```python
from build123d import *

# Parameters (mm, degrees)
SKETCH_1_W           = 46
SKETCH_1_H           = 30
EXTRUDE_1_DEPTH      = 3.5
SKETCH_2_W           = 46
SKETCH_2_H           = 5
EXTRUDE_2_DEPTH      = 33.5
SKETCH_4_R           = 1.3
CUT_EXTRUDE_2_DEPTH  = 15
SKETCH_5_R           = 1.3
CUT_EXTRUDE_3_DEPTH  = 15
CUT_EXTRUDE_4_REACH  = 49.71
SKETCH_6_W           = 5
SKETCH_6_H           = 3.7
SKETCH_7_W           = 46
SKETCH_7_H           = 25
EXTRUDE_3_DEPTH      = 15
SKETCH_8_W           = 46
SKETCH_8_H           = 2
CUT_EXTRUDE_5_DEPTH  = 14
SKETCH_10_W          = 5
SKETCH_10_H          = 3.7
CUT_EXTRUDE_7_DEPTH  = 5
FILLET_1_R           = 6
FILLET_2_R           = 4
SKETCH_11_W          = 5
SKETCH_11_H          = 23.135705429
CUT_EXTRUDE_8_DEPTH  = 14
FILLET_3_R           = 4
FILLET_4_R           = 1
SKETCH_12_W          = 1.2
SKETCH_12_H          = 0.5
EXTRUDE_4_DEPTH      = 10
SKETCH_13_W          = 1.2
SKETCH_13_H          = 0.5
EXTRUDE_5_DEPTH      = 10
SKETCH_14_W          = 57.080352076
SKETCH_14_H          = 14
CUT_EXTRUDE_9_DEPTH  = 2.5
FILLET_5_R           = 4
SKETCH_15_R          = 1.3
CUT_EXTRUDE_10_DEPTH = 8
SKETCH_16_W          = 5
SKETCH_16_H          = 1.8
CUT_EXTRUDE_11_DEPTH = 7
SKETCH_17_W          = 5
SKETCH_17_H          = 1.8
CUT_EXTRUDE_12_DEPTH = 7
SKETCH_18_R          = 3
CUT_EXTRUDE_13_DEPTH = 4


with BuildPart() as part:
    # Эскиз1 → Бобышка-Вытянуть1 (new body)
    with BuildSketch(Plane.XY):
        Rectangle(SKETCH_1_W, SKETCH_1_H)
    extrude(amount=EXTRUDE_1_DEPTH)

    # Эскиз2 → Бобышка-Вытянуть2 (add)
    with BuildSketch(Plane(origin=(0, 0, 0), x_dir=(-1, 0, 0), z_dir=(0, 0, -1))):
        with Locations((0, -12.5)):
            Rectangle(SKETCH_2_W, SKETCH_2_H)
    extrude(amount=EXTRUDE_2_DEPTH)

    # Эскиз4 → Вырез-Вытянуть2 (cut)
    with BuildSketch(Plane(origin=(0, 15, 0), x_dir=(1, 0, 0), z_dir=(0, 1, 0))):
        with Locations(Location((15, -1.5, 0), (0, 0, 270))):
            Circle(SKETCH_4_R)
        with Locations(Location((-15, -1.5, 0), (0, 0, 270))):
            Circle(SKETCH_4_R)
    extrude(amount=-CUT_EXTRUDE_2_DEPTH, mode=Mode.SUBTRACT)

    # Эскиз5 → Вырез-Вытянуть3 (cut)
    with BuildSketch(Plane(origin=(0, 0, -33.5), x_dir=(-1, 0, 0), z_dir=(0, 0, -1))):
        with Locations((-20, -12.5)):
            Circle(SKETCH_5_R)
        with Locations((20, -12.5)):
            Circle(SKETCH_5_R)
    extrude(amount=-CUT_EXTRUDE_3_DEPTH, mode=Mode.SUBTRACT)

    # Эскиз6 → Вырез-Вытянуть4 (cut, up to next)
    with BuildSketch(Plane(origin=(0, -10, 0), x_dir=(1, 0, 0), z_dir=(0, 1, 0)), mode=Mode.PRIVATE) as cut_extrude_4_sk1:
        with Locations((-15, 25.35)):
            Rectangle(SKETCH_6_W, SKETCH_6_H)
    cut_extrude_4_tool1 = extrude(cut_extrude_4_sk1.sketch, amount=-CUT_EXTRUDE_4_REACH, mode=Mode.PRIVATE) & part.part
    # Эскиз6 → Вырез-Вытянуть4 (cut, up to next)
    with BuildSketch(Plane(origin=(0, -10, 0), x_dir=(1, 0, 0), z_dir=(0, 1, 0)), mode=Mode.PRIVATE) as cut_extrude_4_sk2:
        with Locations((15, 25.35)):
            Rectangle(SKETCH_6_W, SKETCH_6_H)
    cut_extrude_4_tool2 = extrude(cut_extrude_4_sk2.sketch, amount=-CUT_EXTRUDE_4_REACH, mode=Mode.PRIVATE) & part.part
    add(cut_extrude_4_tool1.solids().sort_by_distance((-15, -10, -25.35))[0], mode=Mode.SUBTRACT)
    add(cut_extrude_4_tool2.solids().sort_by_distance((15, -10, -25.35))[0], mode=Mode.SUBTRACT)

    # Эскиз7 → Бобышка-Вытянуть3 (add)
    with BuildSketch(Plane(origin=(0, 0, 0), x_dir=(-1, 0, 0), z_dir=(0, 0, -1))):
        with Locations((0, 2.5)):
            Rectangle(SKETCH_7_W, SKETCH_7_H)
    extrude(amount=EXTRUDE_3_DEPTH)

    # Эскиз8 → Вырез-Вытянуть5 (cut)
    with BuildSketch(Plane(origin=(0, 0, -15), x_dir=(-1, 0, 0), z_dir=(0, 0, -1))):
        with Locations((0, 6.62)):
            Rectangle(SKETCH_8_W, SKETCH_8_H)
        with Locations((0, -1.38)):
            Rectangle(SKETCH_8_W, SKETCH_8_H)
    extrude(amount=-CUT_EXTRUDE_5_DEPTH, mode=Mode.SUBTRACT)

    # Эскиз10 → Вырез-Вытянуть7 (cut)
    with BuildSketch(Plane.XY.offset(3.5)):
        with Locations((15, 6)):
            Rectangle(SKETCH_10_W, SKETCH_10_H)
        with Locations((-15, 6)):
            Rectangle(SKETCH_10_W, SKETCH_10_H)
    extrude(amount=-CUT_EXTRUDE_7_DEPTH, mode=Mode.SUBTRACT)

    # Скругление1
    fillet_1_edges = [part.edges().sort_by_distance(p)[0] for p in [
        (0, -15, 3.5),
    ]]
    fillet(fillet_1_edges, radius=FILLET_1_R)

    # Скругление2
    fillet_2_edges = [part.edges().sort_by_distance(p)[0] for p in [
        (0, -10, -15),
    ]]
    fillet(fillet_2_edges, radius=FILLET_2_R)

    # Эскиз11 → Вырез-Вытянуть8 (cut)
    with BuildSketch(Plane(origin=(0, 0, -15), x_dir=(-1, 0, 0), z_dir=(0, 0, -1))):
        with Locations((0, -5.947852714)):
            Rectangle(SKETCH_11_W, SKETCH_11_H)
    extrude(amount=-CUT_EXTRUDE_8_DEPTH, mode=Mode.SUBTRACT)

    # Скругление3
    # the kernel refuses this fillet: 4 mm, written as the material it takes off along each edge
    with BuildSketch(Plane(origin=(-2.5, 5.62, -25), x_dir=(-1, 0, 0), z_dir=(0, 0, 1))) as fillet_3_piece_1:
        with BuildLine():
            CenterArc((FILLET_3_R, FILLET_3_R), FILLET_3_R, 180, 90)
            Line((0, FILLET_3_R), (0, 0))
            Line((0, 0), (FILLET_3_R, 0))
        make_face()
    extrude(amount=24, mode=Mode.SUBTRACT)
    with BuildSketch(Plane(origin=(-2.5, -2.38, -1), x_dir=(-1, 0, 0), z_dir=(0, 0, -1))) as fillet_3_piece_2:
        with BuildLine():
            CenterArc((FILLET_3_R, -FILLET_3_R), FILLET_3_R, 90, 90)
            Line((0, -FILLET_3_R), (0, 0))
            Line((0, 0), (FILLET_3_R, 0))
        make_face()
    extrude(amount=14, mode=Mode.SUBTRACT)
    with BuildSketch(Plane(origin=(2.5, -2.38, -15), x_dir=(0, -1, 0), z_dir=(0, 0, 1))) as fillet_3_piece_3:
        with BuildLine():
            CenterArc((FILLET_3_R, FILLET_3_R), FILLET_3_R, 180, 90)
            Line((0, FILLET_3_R), (0, 0))
            Line((0, 0), (FILLET_3_R, 0))
        make_face()
    extrude(amount=14, mode=Mode.SUBTRACT)
    with BuildSketch(Plane(origin=(2.5, 5.62, -25), x_dir=(1, 0, 0), z_dir=(0, 0, 1))) as fillet_3_piece_4:
        with BuildLine():
            CenterArc((FILLET_3_R, -FILLET_3_R), FILLET_3_R, 90, 90)
            Line((0, -FILLET_3_R), (0, 0))
            Line((0, 0), (FILLET_3_R, 0))
        make_face()
    extrude(amount=24, mode=Mode.SUBTRACT)

    # Скругление4
    fillet_4_edges = [part.edges().sort_by_distance(p)[0] for p in [
        (-23, 3, 3.5),
        (23, 3, 3.5),
        (23, -15, -18),
        (23, -13.242640687, 1.742640687),
        (-23, -15, -18),
        (-23, -13.242640687, 1.742640687),
    ]]
    fillet(fillet_4_edges, radius=FILLET_4_R)

    # Эскиз12 → Бобышка-Вытянуть4 (add)
    with BuildSketch(Plane(origin=(23, 0, 0), x_dir=(0, 0, -1), z_dir=(1, 0, 0))):
        with Locations((9.6, 5.87)):
            Rectangle(SKETCH_12_W, SKETCH_12_H)
        with Locations((8, -0.63)):
            Rectangle(SKETCH_12_W, SKETCH_12_H)
    extrude(amount=-EXTRUDE_4_DEPTH)

    # Эскиз13 → Бобышка-Вытянуть5 (add)
    with BuildSketch(Plane.ZY.offset(23)):
        with Locations((-8, 5.87)):
            Rectangle(SKETCH_13_W, SKETCH_13_H)
        with Locations((-9.6, -0.63)):
            Rectangle(SKETCH_13_W, SKETCH_13_H)
    extrude(amount=-EXTRUDE_5_DEPTH)

    # Эскиз14 → Вырез-Вытянуть9 (cut)
    with BuildSketch(Plane.XZ.offset(15)):
        with Locations((0, -8)):
            Rectangle(SKETCH_14_W, SKETCH_14_H)
    extrude(amount=-CUT_EXTRUDE_9_DEPTH, mode=Mode.SUBTRACT)

    # Скругление5
    fillet_5_edges = [part.edges().sort_by_distance(p)[0] for p in [
        (-2.5, -12.5, -8),
        (2.5, -12.5, -8),
    ]]
    fillet(fillet_5_edges, radius=FILLET_5_R)

    # Эскиз15 → Вырез-Вытянуть10 (cut)
    with BuildSketch(Plane.XZ.offset(12.5)):
        with Locations(Location((-19, -8, 0), (0, 0, 270))):
            Circle(SKETCH_15_R)
        with Locations(Location((19, -8, 0), (0, 0, 270))):
            Circle(SKETCH_15_R)
    extrude(amount=-CUT_EXTRUDE_10_DEPTH, mode=Mode.SUBTRACT)

    # Эскиз16 → Вырез-Вытянуть11 (cut)
    with BuildSketch(Plane.ZY.offset(23)):
        with Locations((-8, -6.3)):
            Rectangle(SKETCH_16_W, SKETCH_16_H)
    extrude(amount=-CUT_EXTRUDE_11_DEPTH, mode=Mode.SUBTRACT)

    # Эскиз17 → Вырез-Вытянуть12 (cut)
    with BuildSketch(Plane(origin=(23, 0, 0), x_dir=(0, 0, -1), z_dir=(1, 0, 0))):
        with Locations((8, -6.3)):
            Rectangle(SKETCH_17_W, SKETCH_17_H)
    extrude(amount=-CUT_EXTRUDE_12_DEPTH, mode=Mode.SUBTRACT)

    # Эскиз18 → Вырез-Вытянуть13 (cut)
    with BuildSketch(Plane(origin=(0, 15, 0), x_dir=(1, 0, 0), z_dir=(0, 1, 0))):
        with Locations(Location((8, 10, 0), (0, 0, 270))):
            Circle(SKETCH_18_R)
        with Locations(Location((-8, 10, 0), (0, 0, 90))):
            Circle(SKETCH_18_R)
        Polygon((3.75277675, 15.5), (1.876388375, 18.75), (-1.876388375, 18.75), (-3.75277675, 15.5), (-1.876388375, 12.25), (1.876388375, 12.25), align=None)
    extrude(amount=-CUT_EXTRUDE_13_DEPTH, mode=Mode.SUBTRACT)


solid = part.part
```
Can you work these out from the model? Positions are in its coordinate system, mm. A direction names the side the tool comes from. Coordinates: 2 decimals unless noted, no trailing zeros. Loops run counter-clockwise (first coordinate to the right, second up) from the corner with the lowest first, then second, coordinate; pieces in that order, holes last. Notation, with made-up numbers: (-9.5, 80) -> (41.5, 80) arc R20 cw to (41.5, 93) -> close; hole circle Ø9 at (42, 17.5). An arc over 180 degrees is marked (long way). Put each result on its own line as item: value. Start each with the question number.
Q1. I want a section at B-B (x = 8). Write out the boundary of the cut face in (y, z), plus the area to 3 significant figures.
Q2. I want a section at A-A (z = -3). Write out the boundary of the cut face in (x, y), plus the area to 3 significant figures.
Q3. I'm going to push flat-ended pins straight in: P1, Ø6, axis at x = 3, y = 0.5, coming from the -Z side; P2, Ø0.6, axis at x = 17.5, z = -8, coming from the -Y side; P3, Ø3, axis at y = 7, z = -17, coming from the +X side; P4, Ø2, axis at x = -0.5, y = 12.5, coming from the -Z side. Where does each tip first touch, or does it pass through?
Q4. If I drill on line 1 (X direction, y = 1.1, z = 1.5); line 2 (Y direction, x = 11.5, z = -3.5); line 3 (X direction, y = -8.65, z = -8), over which ranges is the centre line in solid material (lowest first)? Write a range as [from, to].
Q5. Thinking about a two-plate mould opening in X: for faces 6 (the face through (-13, -4, -15)), 7 (the face through (3.703, 4.479, -8.098)), 8 (the face through (-22.699, -14.715, -24.12)), which applies, pulls with the +X half, pulls with the -X half, needs draft (parallel to the pull), parting line crosses it, or undercut?
Q6. For faces 1 (the face through (-13, 3, -15)), 2 (the face through (-20, -6, -5.5)), 3 (the face through (-20, -12, -18.5)), 4 (the face through (12.5, 6, 1)), 5 (the face through (18.5, -5, -9.2)), which set-ups out of +Z, -Z, +X, -X, +Y, -Y let a thin tool reach every point of the face, with its end or its side?
Q7. I want a section at C-C (x = 15). Count the separate pieces of the cut face and the enclosed holes in it, plus the area to 3 significant figures.
Q8. I want a section at D-D (y = 5). Write out the boundary of the cut face in (x, z), plus the area to 3 significant figures.
Taken from the geometry:
1. outline: (-15, -33.5) -> (-10, -33.5) -> (-10, -19) arc R4 cw to (-6, -15) -> (-2.38, -15) -> (-2.38, -1) -> (-0.38, -1) -> (-0.38, -15) -> (5.62, -15) -> (5.62, -1) -> (7.62, -1) -> (7.62, -15) -> (15, -15) -> (15, -13) -> (11, -13) -> (11, -7) -> (15, -7) -> (15, 3.5) -> (-9, 3.5) arc R6 ccw to (-14.81, -1) -> (-12.5, -1) -> (-12.5, -15) -> (-15, -15) -> close
1. area: 528 mm2
2. outline: (-23, -12.5) -> (-6.5, -12.5) arc R4 ccw to (-2.5, -8.5) -> (-2.5, -6.38) arc R4 ccw to (-6.5, -2.38) -> (-23, -2.38) -> close; (-23, -0.38) -> (-2.5, -0.38) -> (-2.5, 1.62) arc R4 ccw to (-6.5, 5.62) -> (-23, 5.62) -> close; (-23, 7.62) -> (23, 7.62) -> (23, 15) -> (-23, 15) -> close; (2.5, -8.5) arc R4 ccw to (6.5, -12.5) -> (23, -12.5) -> (23, -2.38) -> (6.5, -2.38) arc R4 ccw to (2.5, -6.38) -> close; (2.5, -0.38) -> (23, -0.38) -> (23, 5.62) -> (6.5, 5.62) arc R4 ccw to (2.5, 1.62) -> close
2. area: 980 mm2
3. P1: stops at z = -15
3. P2: stops at y = -12.5
3. P3: passes through
3. P4: stops at z = -12.25
4. line 1: x = [-23, -16.3], [-13.7, 13.7], [16.3, 23]
4. line 2: y = [-12.5, -2.38], [-0.38, 5.62], [7.62, 15]
4. line 3: x = [-23, -20.3], [-17.7, -2.5], [2.5, 17.7], [20.3, 23]
5. face 6: needs draft
5. face 7: undercut
5. face 8: pulls with the -X half
6. face 1: -Z, +X, -X, +Y
6. face 2: -X
6. face 3: -Z
6. face 4: +Z
6. face 5: -Y
7. separate pieces: 4
7. enclosed holes: 0
7. area: 488 mm2
8. outline: (-23, -15) -> (-4.36, -15) -> (-4.36, -1) -> (4.36, -1) -> (4.36, -15) -> (23, -15) -> (23, 2.5) arc R1 ccw to (22, 3.5) -> (17.5, 3.5) -> (17.5, -1.5) -> (12.5, -1.5) -> (12.5, 3.5) -> (-12.5, 3.5) -> (-12.5, -1.5) -> (-17.5, -1.5) -> (-17.5, 3.5) -> (-22, 3.5) arc R1 ccw to (-23, 2.5) -> close
8. area: 678 mm2
